```python
from build123d import *

# Parameters (mm, degrees)
BOSS_EXTRUDE1_DEPTH = 5
SKETCH4_R           = 2.15
BOSS_EXTRUDE2_DEPTH = 5


with BuildPart() as part:
    # Sketch3 → Boss-Extrude1 (new body)
    with BuildSketch(Plane.XY):
        with BuildLine():
            ThreePointArc((16.161070517, 9.296643019), (-1.117119854, 14.203399989), (-7.139484482, -2.718279914))
            add(Edge.make_bspline(
                [(-7.139484482, -2.718279914), (9.132754629, -50.436524862), (33.087399733, -95.298268059), (61.843065412, -136.60626672)],
                knots=[0, 0, 0, 0, 1, 1, 1, 1], degree=3))
            ThreePointArc((61.843065412, -136.60626672), (79.680701211, -142.48791497), (85.233269402, -124.545116316))
            add(Edge.make_bspline(
                [(16.161070517, 9.296643019), (45.599741143, -31.632336181), (68.256168937, -77.163504674), (85.233269402, -124.545116316)],
                knots=[0, 0, 0, 0, 1, 1, 1, 1], degree=3))
        make_face()
        Polygon((78.262696046, -131.010190899), (76.145869285, -126.905026127), (71.532278927, -126.685669492), (69.035515328, -130.571477627), (71.152342089, -134.676642399), (75.765932447, -134.895999034), align=None, mode=Mode.SUBTRACT)
        Polygon((55.347374171, -86.570478665), (53.230547411, -82.465313894), (48.616957052, -82.245957258), (46.120193454, -86.131765394), (48.237020214, -90.236930165), (52.850610573, -90.456286801), align=None, mode=Mode.SUBTRACT)
        Polygon((32.432052297, -42.130766432), (30.315225536, -38.025601661), (25.701635178, -37.806245025), (23.204871579, -41.69205316), (25.32169834, -45.797217932), (29.935288698, -46.016574567), align=None, mode=Mode.SUBTRACT)
        Polygon((9.516730422, 2.308945802), (7.399903662, 6.414110573), (2.786313303, 6.633467209), (0.289549705, 2.747659073), (2.406376465, -1.357505698), (7.019966824, -1.576862334), align=None, mode=Mode.SUBTRACT)
    extrude(amount=BOSS_EXTRUDE1_DEPTH)

    # Sketch4 → Boss-Extrude2 (add)
    # profile 1 of 2: a face of its own
    with BuildSketch(Plane.XY.offset(5)):
        with BuildLine():
            Line((-62.450693281, -97.22736689), (15.220358234, -57.176316709))
            add(Edge.make_bspline(
                [(2.997808313, -29.725276343), (6.797307694, -38.99575652), (10.8790517, -48.14793286), (15.220358234, -57.176316709)],
                knots=[0.19087071, 0.19087071, 0.19087071, 0.19087071, 0.389797815, 0.389797815, 0.389797815, 0.389797815], degree=3))
            Line((2.997808313, -29.725276343), (-68.216036929, -66.446670398))
            add(Edge.make_bspline(
                [(-77.409704675, -65.483914752), (-72.739634543, -62.850222111), (-68.216036929, -66.446670398)],
                knots=[0, 0, 0, 1, 1, 1], degree=2))
            Line((-77.409704675, -65.483914752), (-80.411912193, -67.033578992))
            Line((-80.411912193, -67.033578992), (-78.087434927, -71.536853276))
            add(Edge.make_bspline(
                [(-79.1174503, -76.560041992), (-76.157677443, -74.63824268), (-78.087434927, -71.536853276)],
                knots=[0.011104225, 0.011104225, 0.011104225, 1, 1, 1], degree=2))
            add(Edge.make_bspline(
                [(-76.835042304, -78.059565803), (-77.986988957, -77.094288184), (-79.1174503, -76.560041992)],
                knots=[0, 0, 0, 1, 1, 1], degree=2))
            Line((-76.835042304, -78.059565803), (-67.839096009, -95.50541566))
            ThreePointArc((-67.839096009, -95.50541566), (-65.501522422, -97.48236602), (-62.450693281, -97.22736689))
        make_face()
        with Locations((-58.886757215, -87.65648791)):
            Circle(SKETCH4_R, mode=Mode.SUBTRACT)
        with Locations((-65.092650278, -75.633639142)):
            Circle(SKETCH4_R, mode=Mode.SUBTRACT)
    # profile 2 of 2: a face of its own
    with BuildSketch(Plane.XY.offset(5)):
        with BuildLine():
            add(Edge.make_bspline(
                [(32.280750269, -14.617843465), (37.629854463, -23.089001057), (42.718912178, -31.721489708), (47.556604904, -40.493649318)],
                knots=[0.190825277, 0.190825277, 0.190825277, 0.190825277, 0.38974783, 0.38974783, 0.38974783, 0.38974783], degree=3))
            Line((47.556604904, -40.493649318), (125.205794469, -0.413084682))
            ThreePointArc((125.205794469, -0.413084682), (127.181774896, 1.925308859), (126.925510125, 4.976031949))
            Line((126.925510125, 4.976031949), (117.922327039, 22.418148257))
            add(Edge.make_bspline(
                [(117.922327039, 22.418148257), (117.803338747, 23.916341756), (118.02315462, 25.147212514)],
                knots=[0, 0, 0, 1, 1, 1], degree=2))
            add(Edge.make_bspline(
                [(118.02315462, 25.147212514), (114.741637832, 23.849053997), (113.332685388, 27.219133104)],
                knots=[0.011104225, 0.011104225, 0.011104225, 1, 1, 1], degree=2))
            Line((113.332685388, 27.219133104), (111.010076543, 31.723371329))
            Line((111.010076543, 31.723371329), (108.007226392, 30.174952712))
            add(Edge.make_bspline(
                [(108.007226392, 30.174952712), (103.154331871, 27.895631161), (103.463399948, 22.124855428)],
                knots=[0, 0, 0, 1, 1, 1], degree=2))
            Line((103.463399948, 22.124855428), (32.280750269, -14.617843465))
        make_face()
        with Locations((115.340727562, 2.229607059)):
            Circle(SKETCH4_R, mode=Mode.SUBTRACT)
        with Locations((109.139822812, 14.255029359)):
            Circle(SKETCH4_R, mode=Mode.SUBTRACT)
    extrude(amount=-BOSS_EXTRUDE2_DEPTH)


solid = part.part
```
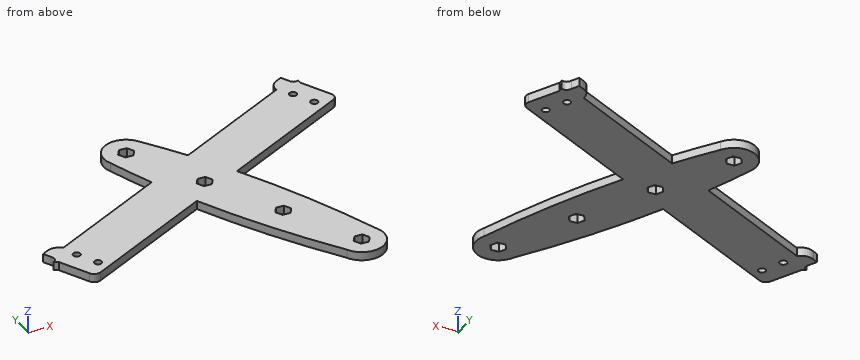
Geometry check sheet. Reference: the model listing, model coordinates, mm. Coordinates: 2 decimals unless noted, no trailing zeros. Write each loop counter-clockwise with the first axis right and the second up, starting at its lowest first coordinate (ties: lowest second). Pieces come first, ordered by that corner, then holes. Notation, with made-up numbers: M 85.25,-29 L 140.25,-29 A33 cw 140.25,8 Z; hole C 81.25,42.25 d2. An arc over 180 degrees is marked long. Use one line per item in the form item = value. Start each with the question number.
1) Thickness scan on probe 1 along Y at (x, z) = (53, 1.15); probe 2 along X at (y, z) = (-75, 3.3); probe 3 along X at (y, z) = (11, 1.1). Record the ranges inside material, lowest first. Write a range as from..to.
2) Section check B-B on x = -26. Enter the section's corners in (y, z), and give its area (3 significant figures).
3) Section check A-A on z = 3.7. State how many separate pieces and enclosed holes the cut face has, and give its area (3 significant figures).
4) Go/stop test with flat-tipped pins: pin 1 Ø2 at (y, z) = (-91, 2.5) entering from -X; pin 2 Ø3 at (y, z) = (-83, 1.5) entering from +X; pin 3 Ø3 at (y, z) = (-107, 2) entering from -X. Record where each tip stops, or that it passes through.
Responses:
q1.probe_1 = -123.56..-90.22, -82.45..-50.62, -37.68..-3.92
q1.probe_2 = -77.61..-67.15, -63.04..-19.35, 24.21..65
q1.probe_3 = -5.14..14.94, 81.91..123.82
q2.outline = M -78.43,0 L -44.68,0 L -44.68,5 L -78.43,5 Z
q2.area = 169 mm2
q3.separate_pieces = 1
q3.enclosed_holes = 8
q3.area = 10,900 mm2
q4.pin_1 = -70.68
q4.pin_2 = 69.29
q4.pin_3 = 41.54
